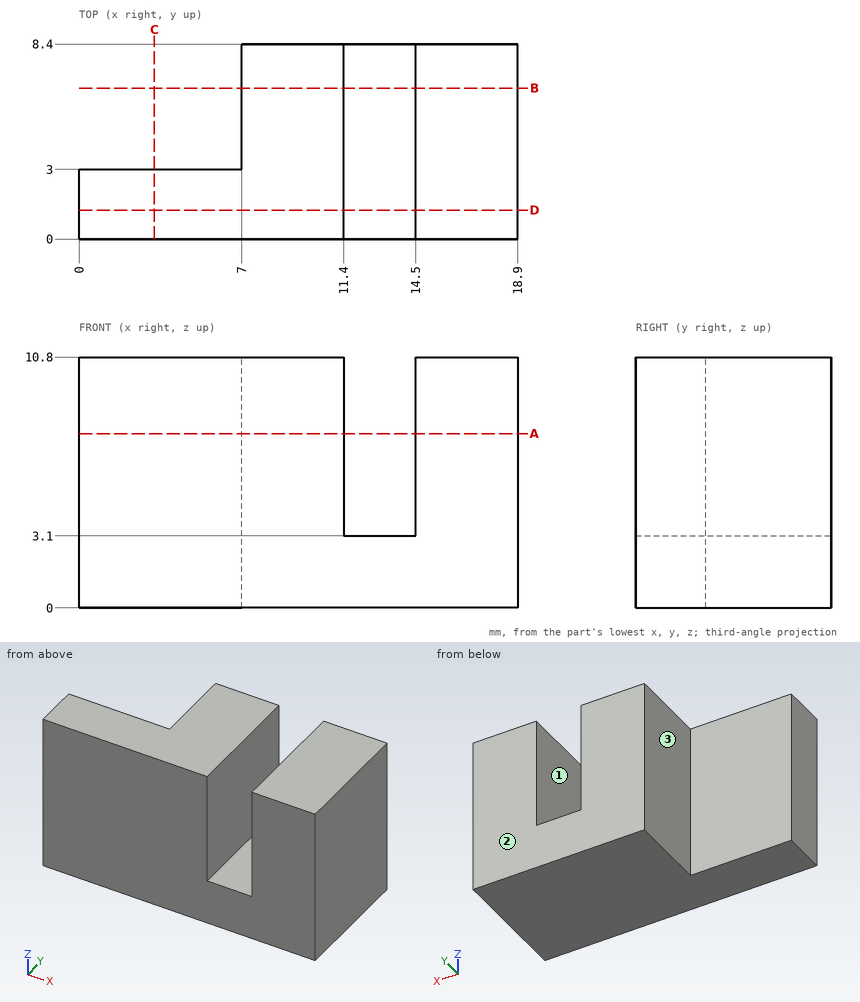
Could you check a few things on this drawing? It's one solid part, dimensions in mm from its lowest x, y, z. A direction names the side the tool comes from. Give positions to 0.01 mm unless a question says otherwise; leave off trailing zeros. Write each loop counter-clockwise with the first axis right and the second up, starting at its lowest first coordinate (ties: lowest second). Pieces come first, ordered by that corner, then holes. Notation, with made-up numbers: M -29.75,76 L -0.75,76 A9 ccw -0.75,93 Z; hole C -3,-2.75 d3. An arc over 180 degrees is marked long. Put each result on its own line as item: value. Start each with the question number.
Item 1: If we section it at C-C, the plane x = 3.25: Write out the boundary of the cut face in (y, z), then the cut area to 3 significant figures.
Item 2: If we section it at D-D, the plane y = 1.25: Write out the boundary of the cut face in (x, z).
Item 3: On a 3-axis mill with a long thin cutter (end or side, diameter ignored), from which of +Z, -Z, +X, -X, +Y, -Y can I reach the whole of each face in a straight line? I mean the marked faces 1, 2 and 3. Say none if no direction works.
Item 4: If we section it at B-B, the plane y = 6.5: Write out the boundary of the cut face in (x, z), then the cut area to 3 significant figures.
Item 5: Will these pins go through, and if not, where does the flat tip stop? pin 1 (3 mm diameter, centred on y = 7, z = 4.5, fed in from -X); pin 2 (5.5 mm diameter, centred on x = 2, z = 4.5, fed in from +Y).
Item 6: If we section it at A-A, the plane z = 7.5: Write out the boundary of the cut face in (x, y).
Item 7: I need wall thicknesses on L1, parallel to X at y = 1.5, z = 9; L2, parallel to X at y = 7, z = 6.5; L3, parallel to Z at x = 12.5, y = 6. Which ranges of each line are inside material? Lowest first, please. Write a range as from..to.
Values:
1. outline: M 0,0 L 3,0 L 3,10.8 L 0,10.8 Z
1. area: 32.4 mm²
2. outline: M 0,0 L 18.9,0 L 18.9,10.8 L 14.5,10.8 L 14.5,3.1 L 11.4,3.1 L 11.4,10.8 L 0,10.8 Z
3. face 1: +Z, +Y, -Y
3. face 2: +Z, -Z, +X, -X, +Y
3. face 3: +Z, -Z, -X, +Y
4. outline: M 7,0 L 18.9,0 L 18.9,10.8 L 14.5,10.8 L 14.5,3.1 L 11.4,3.1 L 11.4,10.8 L 7,10.8 Z
4. area: 105 mm²
5. pin 1: x = 7
5. pin 2: y = 3
6. outline: M 0,0 L 11.4,0 L 11.4,8.4 L 7,8.4 L 7,3 L 0,3 Z; M 14.5,0 L 18.9,0 L 18.9,8.4 L 14.5,8.4 Z
7. L1: 0..11.4, 14.5..18.9
7. L2: 7..11.4, 14.5..18.9
7. L3: 0..3.1
